Autodesk Fusion 360 part; units mm, degrees
sketch "Sketch1" plane through (0, 0, 0) normal (0, 0, 1) x (1, 0, 0) in component "part 1"
  line L0 (-15.5, 12.25) -> (15.5, 12.25)
  line L1 (15.5, 12.25) -> (15.5, -12.25)
  line L2 (15.5, -12.25) -> (-15.5, -12.25)
  line L3 (-15.5, -12.25) -> (-15.5, 12.25)
  line L4 (-15.5, 12.25) -> (15.5, -12.25) construction
  line L5 (15.5, 12.25) -> (-15.5, -12.25) construction
  dimension "d1" = 31
  dimension "d2" = 24.5
extrude "Extrude1" add sketch "Sketch1" along normal blind 6.3 in component "part 1"
sketch "Sketch2" plane through (0, 0, 6.3) normal (0, 0, 1) x (-1, 0, 0) in component "part 1"
  line L0 (15.5, 12.25) -> (-15.5, 12.25)
  line L1 (-15.5, 12.25) -> (-15.5, -12.25)
  line L2 (-15.5, -12.25) -> (15.5, -12.25)
  line L3 (15.5, -12.25) -> (15.5, 12.25)
shell "Shell1" thickness 1.8 removed faces 1 at (-5.1667, 4.0833, 6.3) in component "part 1"
sketch "Sketch3" plane through (0, 0, 6.3) normal (0, 0, 1) x (-1, 0, 0) in component "part 1"
  circle A0 centre (14.4, -11.2) radius 0.85
  line L0 (0, 0) -> (0, -3.5)
  line L1 (0, 0) -> (3.5, 0)
  circle A1 centre (-14.4, -11.2) radius 0.85
  circle A2 centre (-14.4, 11.2) radius 0.85
  circle A3 centre (14.4, 11.2) radius 0.85
  dimension "d8" = 1.7
  dimension "d9" = 11.2
  dimension "d10" = 14.4
extrude "Extrude2" cut sketch "Sketch3" against normal blind 4 in component "part 1"
fillet "Fillet1" radius 1 1 edges at (15.5, -12.25, 3.15) in component "part 1"
fillet "Fillet1" radius 1 1 edges at (15.5, 12.25, 3.15) in component "part 1"
fillet "Fillet1" radius 1 1 edges at (-15.5, 12.25, 3.15) in component "part 1"
fillet "Fillet1" radius 1 1 edges at (-15.5, -12.25, 3.15) in component "part 1"
fillet "Fillet2" radius 0.75 8 edges at (-15.2071, -11.9571, 0) (-15.5, 0, 0) (-15.2071, 11.9571, 0) (0, 12.25, 0) (15.2071, 11.9571, 0) (15.5, 0, 0) (15.2071, -11.9571, 0) (0, -12.25, 0) in component "part 1"
component "part 1" placed x (1, 0, 0) y (0, 1, 0) z (0, 0, 1) at (0, 0, 0)
Work out the finished part from the listing and answer in its coordinate system (mm). A direction names the side the tool comes from. Round coordinates to 2 decimals unless told otherwise and drop trailing zeros. Write each loop counter-clockwise with the first axis right and the second up, starting at its lowest first coordinate (ties: lowest second). Pieces come first, ordered by that corner, then holes. Notation, with made-up numbers: (14.25, 29.5) -> (28.25, 29.5) arc R25 ccw to (28.25, 55.5) -> close; hole circle Ø9 at (-39, 44.5). An arc over 180 degrees is marked (long way). Answer as CSV lines item,"result". Start each with the question number.
(1) Find the intervals of material crossed by probe 1 along Y at (x, z) = (-14.4, 3.85); probe 2 along X at (y, z) = (11.2, 3.25); probe 3 along Y at (x, z) = (13.5, 5), in increasing order.
(2) The part is cut by section A-A, the plane z = 3.75. Give the vertices of the cut face in (x, y), then the cut area to 3 significant figures.
(3) Each of these flat-tipped pins is pushed along its axis until it touches: pin 1 (10.5 mm diameter, centred on x = 2.5, y = 4.5, fed in from +Z); pin 2 (0.5 mm diameter, centred on x = -14.5, y = 11, fed in from +Z). Where does it stop, or does it pass through?
(4) The mould has two halves that part along X. Classify faces 3 (the flat face through (0, 0, 1.8)), 4 (the flat face through (0, 11, 6.3)), 5 (the flat face through (-15.5, 0, 3)): +X half, -X half, draft (parallel to the pull), parting line (faces both ways), or undercut.
(5) A tool of negligible diameter and unlimited length cuts with its end or side. For faces 1 (the flat face through (0, 12.25, 3)), 2 (the flat face through (14, 11, 2.3)), from which of +Z, -Z, +X, -X, +Y, -Y can it reach the whole face along a straight path? Write none if from no direction.
(6) The part is cut by section C-C, the plane x = 11.5. Give the vertices of the cut face in (y, z).
(7) The part is cut by section B-B, the plane y = -1.25. Give the vertices of the cut face in (x, z).
Output values:
1,probe 1,"y = -12.25 to -12.05, -10.35 to 10.35, 12.05 to 12.25"
1,probe 2,"x = -15.5 to -15.25, -13.55 to 13.55, 15.25 to 15.5"
1,probe 3,"y = -12.25 to -10.45, 10.45 to 12.25"
2,outline,"(-15.5, -11.25) arc R1 ccw to (-14.5, -12.25) -> (14.5, -12.25) arc R1 ccw to (15.5, -11.25) -> (15.5, 11.25) arc R1 ccw to (14.5, 12.25) -> (-14.5, 12.25) arc R1 ccw to (-15.5, 11.25) -> close; hole circle Ø1.7 at (-14.4, -11.2); hole circle Ø1.7 at (-14.4, 11.2); hole (-13.7, -10.45) -> (13.7, -10.45) -> (13.7, 10.45) -> (-13.7, 10.45) -> close; hole circle Ø1.7 at (14.4, -11.2); hole circle Ø1.7 at (14.4, 11.2)"
2,area,"177 mm²"
3,pin 1,"stops at z = 1.8"
3,pin 2,"stops at z = 2.3"
4,face 3,"undercut"
4,face 4,"draft"
4,face 5,"-X half"
5,face 1,"+Z, -Z, +X, -X, +Y"
5,face 2,"+Z"
6,outline,"(-12.25, 0.75) arc R0.75 ccw to (-11.5, 0) -> (11.5, 0) arc R0.75 ccw to (12.25, 0.75) -> (12.25, 6.3) -> (10.45, 6.3) -> (10.45, 1.8) -> (-10.45, 1.8) -> (-10.45, 6.3) -> (-12.25, 6.3) -> close"
7,outline,"(-15.5, 0.75) arc R0.75 ccw to (-14.75, 0) -> (14.75, 0) arc R0.75 ccw to (15.5, 0.75) -> (15.5, 6.3) -> (13.7, 6.3) -> (13.7, 1.8) -> (-13.7, 1.8) -> (-13.7, 6.3) -> (-15.5, 6.3) -> close"
